```python
from build123d import *


with BuildPart() as part:
    # Sketch1 → Revolve1 (revolve)
    with BuildSketch(Plane.XY):
        with BuildLine():
            ThreePointArc((-9.310840107, 19.331058169), (-4.730423414, 18.075866931), (0, 17.653))
            ThreePointArc((0, 17.653), (0.898160183, 17.712068298), (1.780848569, 17.888255676))
            Line((1.780848569, 17.888255676), (90.17, 41.656))
            Line((90.17, 41.656), (-59.69, 38.1))
            Line((-59.69, 38.1), (-9.310840107, 19.331058169))
        make_face()
    revolve(axis=Axis((0, 0, 0), (-1, 0, 0)))

    # Sketch2 → Cut-Revolve1 (revolve, cut)
    with BuildSketch(Plane.XY):
        Polygon((-29.085538438, 35.56), (25.4, 31.75), (25.4, 0), (94.515783367, 0), (94.515783367, 51.74538216), (-80.408492958, 51.74538216), (-80.408492958, 0), (-50.8, 0), (-50.8, 31.75), (-42.645476755, 31.75), (-42.645476755, 35.56), align=None)
    revolve(axis=Axis((-50.8, 0, 0), (1, 0, 0)), mode=Mode.SUBTRACT)


solid = part.part
```
Could you check a few things on this model? Use its own coordinates, in mm. Give positions to 0.01 mm unless a question says otherwise; leave off trailing zeros. Write each loop counter-clockwise with the first axis right and the second up, starting at its lowest first coordinate (ties: lowest second). Pieces come first, ordered by that corner, then holes. Notation, with made-up numbers: (-31, 67) - (6, 67) arc R35 cw to (6, 102) - close; hole circle Ø3 at (33.25, 68.5). An arc over 180 degrees is marked (long way). One line per item, written item: value. Start each with the question number.
Item 1: Imagine slicing it at D-D, the plane x = -37.5. List the corners of the cut face in (y, z) for me, and give its area (3 significant figures).
Item 2: I'm going to push flat-ended pins straight in: pin 1 (1.5 mm diameter, centred on x = 1.5, y = -11.5, fed in from -Z); pin 2 (2 mm diameter, centred on x = -18, z = -6.5, fed in from -Y); pin 3 (8 mm diameter, centred on x = -25, y = 11, fed in from +Z). Where does each tip first touch, or does it pass through?
Item 3: Please list where these lines run through material, in increasing order: line 1 (Z direction, x = -35, y = 11); line 2 (Y direction, x = 11.5, z = 16.5); line 3 (Z direction, x = -21, y = 4). Write a range as from..to.
Item 4: If we mould it in two halves opening along Y, with no side actions, what happens to faces 1 (the face through (-18.337, -2.954, -22.501)), 2 (the face through (25.4, -7.2, -23.4)), 3 (the face through (-35.771, -7.709, -34.714))? For each: +Y half, -Y half, draft (parallel to the pull), parting line (faces both ways), or undercut.
Item 5: Imagine slicing it at C-C, the plane x = 5. List the corners of the cut face in (y, z) for me, and give its area (3 significant figures).
Item 6: Imagine slicing it at A-A, the plane y = 0. List the corners of the cut face in (x, z) for me.
Geometry says:
1. outline: circle Ø71.12 at (0, 0); hole circle Ø59.67 at (0, 0)
1. area: 1,180 mm^2
2. pin 1: z = -31.65
2. pin 2: y = -34.36
2. pin 3: z = 34.62
3. line 1: -33.82..-26.73, 26.73..33.82
3. line 2: -28.26..-12.17, 12.17..28.26
3. line 3: -34.77..-23.35, 23.35..34.77
4. face 1: undercut
4. face 2: draft
4. face 3: parting line
5. outline: circle Ø66.35 at (0, 0); hole circle Ø37.51 at (0, 0)
5. area: 2,350 mm^2
6. outline: (-42.65, -35.56) - (-29.09, -35.56) - (25.4, -31.75) - (25.4, -24.24) - (1.78, -17.89) arc R6.86 ccw to (0, -17.65) arc R26.67 ccw to (-9.31, -19.33) - (-42.65, -31.75) - close; (-42.65, 31.75) - (-9.31, 19.33) arc R26.67 ccw to (0, 17.65) arc R6.86 ccw to (1.78, 17.89) - (25.4, 24.24) - (25.4, 31.75) - (-29.09, 35.56) - (-42.65, 35.56) - close
